Geometry check sheet. Reference: the model listing, model coordinates, mm. Face numbers are marked on the shaded views. A direction names the side the tool comes from. Round coordinates to 2 decimals unless told otherwise and drop trailing zeros. Loops run counter-clockwise (first coordinate to the right, second up) from the corner with the lowest first, then second, coordinate; pieces in that order, holes last. Notation, with made-up numbers: M -16.75,-23.5 L 10.25,-23.5 A29 cw 10.25,-0.5 Z; hole C 68.5,33 d6. An arc over 180 degrees is marked long. Write item = value, one per line.
from build123d import *
from OCP.BRepFilletAPI import BRepFilletAPI_MakeChamfer

# Parameters (mm, degrees)
EXTRUDE_1_DEPTH  = 20
CHAMFER_1_SIZE   = 0.5
EXTRUDE_2_DEPTH  = 20
CHAMFER_3_SIZE   = 1.37373871
CHAMFER_3_SIZE_2 = 0.5
CHAMFER_4_SIZE   = 0.5


with BuildPart() as part:
    # 草图1 → 凸台-拉伸1 (new body)
    with BuildSketch(Plane.XY):
        Polygon((2.309401077, 0), (1.154700538, 2), (-1.154700538, 2), (-2.309401077, 0), (-1.154700538, -2), (1.154700538, -2), align=None)
    extrude(amount=EXTRUDE_1_DEPTH)

    # 倒角1
    chamfer_1_edges = [part.edges().sort_by_distance(p)[0] for p in [
        (0, 2, 20),
        (-1.732050808, 1, 20),
        (-1.732050808, -1, 20),
        (0, -2, 20),
        (1.732050808, -1, 20),
        (1.732050808, 1, 20),
    ]]
    chamfer(chamfer_1_edges, length=CHAMFER_1_SIZE)

    # 草图2 → 凸台-拉伸2 (add)
    with BuildSketch(Plane(origin=(0, 0, 0), x_dir=(-1, 0, 0), z_dir=(0, 0, -1))):
        Polygon((2.886751346, 0), (1.443375673, 2.5), (-1.443375673, 2.5), (-2.886751346, 0), (-1.443375673, -2.5), (1.443375673, -2.5), align=None)
    extrude(amount=EXTRUDE_2_DEPTH)

    # 倒角3
    chamfer_3_edges_1 = [part.edges().sort_by_distance(p)[0] for p in [
        (-2.165063509, -1.25, 0),
    ]]
    chamfer_3_side_1 = [part.faces().sort_by_distance(p)[0] for p in [
        (-2.165063509, -1.25, -0.01),
    ]]
    chamfer_3_edges_2 = [part.edges().sort_by_distance(p)[0] for p in [
        (-2.165063509, 1.25, 0),
    ]]
    chamfer_3_side_2 = [part.faces().sort_by_distance(p)[0] for p in [
        (-2.165063509, 1.25, -0.01),
    ]]
    chamfer_3_edges_3 = [part.edges().sort_by_distance(p)[0] for p in [
        (0, 2.5, 0),
    ]]
    chamfer_3_side_3 = [part.faces().sort_by_distance(p)[0] for p in [
        (0, 2.5, -0.01),
    ]]
    chamfer_3_edges_4 = [part.edges().sort_by_distance(p)[0] for p in [
        (2.165063509, 1.25, 0),
    ]]
    chamfer_3_side_4 = [part.faces().sort_by_distance(p)[0] for p in [
        (2.156403255, 1.245, 0),
    ]]
    chamfer_3_edges_5 = [part.edges().sort_by_distance(p)[0] for p in [
        (2.165063509, -1.25, 0),
    ]]
    chamfer_3_side_5 = [part.faces().sort_by_distance(p)[0] for p in [
        (2.156403255, -1.245, 0),
    ]]
    chamfer_3_edges_6 = [part.edges().sort_by_distance(p)[0] for p in [
        (0, -2.5, 0),
    ]]
    chamfer_3_side_6 = [part.faces().sort_by_distance(p)[0] for p in [
        (0, -2.49, 0),
    ]]
    chamfer_3 = BRepFilletAPI_MakeChamfer(part.part.solid().wrapped)
    for e in chamfer_3_edges_1:
        chamfer_3.Add(CHAMFER_3_SIZE - 0.0001, CHAMFER_3_SIZE_2 - 0.0001, e.wrapped, chamfer_3_side_1[0].wrapped)
    for e in chamfer_3_edges_2:
        chamfer_3.Add(CHAMFER_3_SIZE - 0.0001, CHAMFER_3_SIZE_2 - 0.0001, e.wrapped, chamfer_3_side_2[0].wrapped)
    for e in chamfer_3_edges_3:
        chamfer_3.Add(CHAMFER_3_SIZE - 0.0001, CHAMFER_3_SIZE_2 - 0.0001, e.wrapped, chamfer_3_side_3[0].wrapped)
    for e in chamfer_3_edges_4:
        chamfer_3.Add(CHAMFER_3_SIZE_2 - 0.0001, CHAMFER_3_SIZE - 0.0001, e.wrapped, chamfer_3_side_4[0].wrapped)
    for e in chamfer_3_edges_5:
        chamfer_3.Add(CHAMFER_3_SIZE_2 - 0.0001, CHAMFER_3_SIZE - 0.0001, e.wrapped, chamfer_3_side_5[0].wrapped)
    for e in chamfer_3_edges_6:
        chamfer_3.Add(CHAMFER_3_SIZE_2 - 0.0001, CHAMFER_3_SIZE - 0.0001, e.wrapped, chamfer_3_side_6[0].wrapped)
    add(Compound.cast(chamfer_3.Shape()), mode=Mode.REPLACE)  # a hair under: the kernel refuses the full size

    # 倒角4
    chamfer_4_edges = [part.edges().sort_by_distance(p)[0] for p in [
        (-2.165063509, -1.25, -20),
        (-2.165063509, 1.25, -20),
        (0, 2.5, -20),
        (2.165063509, 1.25, -20),
        (2.165063509, -1.25, -20),
        (0, -2.5, -20),
    ]]
    chamfer(chamfer_4_edges, length=CHAMFER_4_SIZE)


solid = part.part
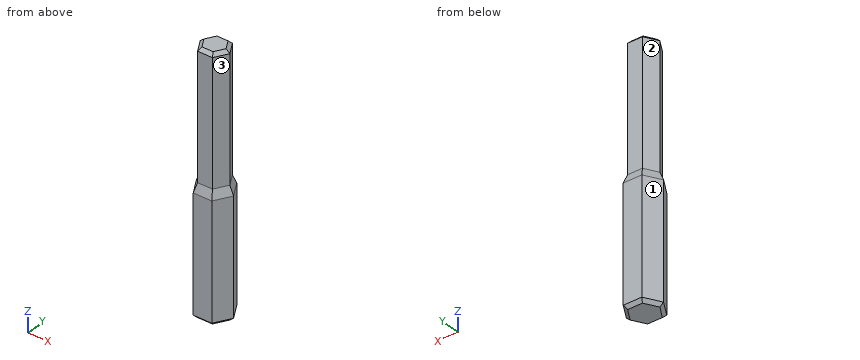
(1) Sectioned sample at A-A on z = -3.5. Record the cut outline in (x, y).
Result set:
outline = M -2.89,0 L -1.44,-2.5 L 1.44,-2.5 L 2.89,0 L 1.44,2.5 L -1.44,2.5 Z
(2) Depth check by flat-ended pin: pin 1 Ø0.7 at (x, z) = (0.5, 9) entering from +Y; pin 2 Ø2 at (y, z) = (-1.5, 0.5) entering from +X; pin 3 Ø2.5 at (x, z) = (0, 6.5) entering from -Y. Enter the tip coordinate at first touch or a pass-through.
Result set:
pin_1 = 2
pin_2 = 2.02
pin_3 = -2
(3) Sectioned sample at C-C on z = 2.5. Record the cut outline in (x, y), then the cut area to 3 significant figures.
Result set:
outline = M -2.31,0 L -1.15,-2 L 1.15,-2 L 2.31,0 L 1.15,2 L -1.15,2 Z
area = 13.9 mm2
(4) Material ranges on line 1 along X through (y, z) = (-1, 18.5); line 2 along Y through (x, z) = (-0.85, 18); line 3 along X through (y, z) = (1.5, -4), recorded low to high. Write a range as from..to.
Result set:
line_1 = -1.73..1.73
line_2 = -2..2
line_3 = -2.02..2.02
(5) Tool access check on the marked faces 1, 2 and 3. Record the directions out of +Z, -Z, +X, -X, +Y, -Y that give a thin tool (end or side, any length) a straight path to the whole face; none if there is none.
Result set:
face_1 = +Z, -Z, -X, +Y
face_2 = +Z, -X, +Y
face_3 = +Z, +X, -Y
